Here's how the part is built. I have some questions about the finished solid (model axes, mm). A direction names the side the tool comes from. Round coordinates to 2 decimals unless told otherwise and drop trailing zeros. Order: outer loops, then holes, each group sorted by start corner. A loop starts at its lowest first (then second) coordinate and runs counter-clockwise, first axis right, second up. Notation, with made-up numbers: (18, -35) -> (43, -35) arc R16 cw to (43, -17) -> close; hole circle Ø1 at (38.5, 83). An arc over 180 degrees is marked (long way). One line per item, written item: value.
```python
from build123d import *

# Parameters (mm, degrees)
SKETCH1_R               = 7.5
BOSS_EXTRUDE1_DEPTH     = 25
FILLET1_R               = 1
SKETCH2_R               = 4.1
CUT_EXTRUDE1_DEPTH      = 8.5
CUT_EXTRUDE1_DEPTH_BACK = 8.5
M5_TAPPED_HOLE1_D       = 4.2
M5_TAPPED_HOLE1_DEPTH   = 11
M5_TAPPED_HOLE1_TIP     = 1.2618073


with BuildPart() as part:
    # Sketch1 → Boss-Extrude1 (new body)
    with BuildSketch(Plane(origin=(0, 0, 0), x_dir=(1, 0, 0), z_dir=(0, 1, 0))):
        Circle(SKETCH1_R)
    extrude(amount=BOSS_EXTRUDE1_DEPTH)

    # Fillet1
    fillet1_edges = [part.edges().sort_by_distance(p)[0] for p in [
        (-7.5, 25, 0),
    ]]
    fillet(fillet1_edges, radius=FILLET1_R)

    # Sketch2 → Cut-Extrude1 (cut, two sides)
    with BuildSketch(Plane.XY) as cut_extrude1_sk:
        with Locations((0, 17)):
            Circle(SKETCH2_R)
    extrude(amount=CUT_EXTRUDE1_DEPTH, mode=Mode.SUBTRACT)
    extrude(cut_extrude1_sk.sketch, amount=-CUT_EXTRUDE1_DEPTH_BACK, mode=Mode.SUBTRACT)

    # M5 Tapped Hole1
    with Locations(Plane(origin=(0, 0, 0), x_dir=(-1, 0, 0), z_dir=(0, -1, 0))):
        with Locations((0, 0)):
            Hole(M5_TAPPED_HOLE1_D / 2, depth=M5_TAPPED_HOLE1_DEPTH)
            with Locations((0, 0, -(M5_TAPPED_HOLE1_DEPTH + M5_TAPPED_HOLE1_TIP / 2))):  # 118° drill point
                Cone(0, M5_TAPPED_HOLE1_D / 2, M5_TAPPED_HOLE1_TIP, mode=Mode.SUBTRACT)


solid = part.part
```
Q1. For P1, Ø1, axis at y = 10, z = -2.5, coming from the +X side; P2, Ø1, axis at y = 7.5, z = 4.5, coming from the +X side; P3, Ø4, axis at x = -4, y = 20.5, coming from the +Z side, each with a flat end and sliding along its axis, tell me the tip position at first contact or that it passes through.
Answers:
P1: x = 7.23
P2: x = 6.34
P3: z = 7.23
Q2. I want a section at C-C on y = 23. Write out the boundary of the cut face in (x, z).
Answers:
outline: circle Ø15 at (0, 0)
Q3. I want a section at B-B on y = 5.5. Write out the boundary of the cut face in (x, z), then the cut area to 3 significant figures.
Answers:
outline: circle Ø15 at (0, 0); hole circle Ø4.2 at (0, 0)
area: 163 mm2
Q4. If we mould it in two halves opening along X, with no side actions, what happens to faces 1 (the face through (-0.35, 12.04, -0.11)), 2 (the face through (7.154, 11.832, -2.253)), 3 (the face through (2, 0, 2))? For each: pulls with the +X half, pulls with the -X half, needs draft (parallel to the pull), parting line crosses it, or undercut.
Answers:
face 1: undercut
face 2: parting line crosses it
face 3: needs draft
Q5. I want a section at A-A on y = 17.75. Write out the boundary of the cut face in (x, z), then the cut area to 3 significant figures.
Answers:
outline: (-4.03, -6.32) -> (-4.03, 6.32) arc R7.5 ccw to start; (4.03, -6.32) arc R7.5 ccw to (4.03, 6.32) -> close
area: 61.9 mm2
Q6. Which directions (+Z, -Z, +X, -X, +Y, -Y) give clear straight access to the entire face, cutting with the end or side of a thin tool? Please do faces 4 (the face through (2.003, 5.577, -0.631)), 5 (the face through (-3.022, 19.771, 0.105)).
Answers:
face 4: -Y
face 5: +Z, -Z
Q7. I need wall thicknesses on line 1 along Z through (x, y) = (0, 3); line 2 along Y through (x, z) = (0, -3.25); line 3 along Y through (x, z) = (0.75, 3.25). Which ranges of each line are inside material? Lowest first, please.
Answers:
line 1: -7.5 to -2.1, 2.1 to 7.5
line 2: 0 to 12.9, 21.1 to 25
line 3: 0 to 12.97, 21.03 to 25
